Design review of the part built by this model. Coordinates are the model's own, in mm. A direction names the side the tool comes from. Coordinates: 2 decimals unless noted, no trailing zeros. Loops run counter-clockwise (first coordinate to the right, second up) from the corner with the lowest first, then second, coordinate; pieces in that order, holes last. Notation, with made-up numbers: (47.25, -30.75) -> (95.25, -30.75) arc R16 cw to (95.25, -7.75) -> close; hole circle Ø1 at (-33.5, -23). An arc over 180 degrees is marked (long way). Answer as a JSON object with one key per item and string values.
```python
from build123d import *

# Parameters (mm, degrees)
SKETCH1_W           = 7.5
SKETCH1_H           = 6
BOSS_EXTRUDE1_DEPTH = 3


with BuildPart() as part:
    # Sketch1 → Boss-Extrude1 (new body)
    with BuildSketch(Plane(origin=(0, 0, 0), x_dir=(1, 0, 0), z_dir=(0, 1, 0))):
        Polygon((0, 0), (0, 25.5), (-7.5, 25.5), (-15, 25.5), (-15, -12.75), (0, -12.75), align=None)
        Polygon((0, -25.5), (0, -12.75), (-15, -12.75), (-15, -25.5), (-7.5, -25.5), align=None)
        Polygon((15, -12.75), (0, -12.75), (0, -25.5), (7.5, -25.5), (15, -25.5), align=None)
        Polygon((7.5, 25.5), (0, 25.5), (0, 0), (0, -12.75), (15, -12.75), (15, 25.5), align=None)
        Polygon((-7.5, 25.5), (0, 25.5), (7.5, 25.5), (7.5, 28.5), (-7.5, 28.5), align=None)
        Polygon((-7.5, 25.5), (0, 25.5), (7.5, 25.5), (7.5, 28.5), (-7.5, 28.5), align=None)
        with Locations((-3.75, -28.5)):
            Rectangle(SKETCH1_W, SKETCH1_H)
        with Locations((3.75, -28.5)):
            Rectangle(SKETCH1_W, SKETCH1_H)
    extrude(amount=BOSS_EXTRUDE1_DEPTH)


solid = part.part
```
1) Add section A-A, the plane y = 1.75. Give the boundary of the cut face in (x, z).
Completed:
{"outline": "(-15, -25.5) -> (-7.5, -25.5) -> (-7.5, -28.5) -> (7.5, -28.5) -> (7.5, -25.5) -> (15, -25.5) -> (15, 25.5) -> (7.5, 25.5) -> (7.5, 31.5) -> (-7.5, 31.5) -> (-7.5, 25.5) -> (-15, 25.5) -> close"}
2) Clearance check with flat-ended pins moving along their axes: pin 1 Ø0.9 at (x, y) = (10.5, 1.5) entering from +Z; pin 2 Ø1.5 at (x, y) = (-12.5, 1.5) entering from -Z; pin 3 Ø0.9 at (y, z) = (2, -26.5) entering from +X. State where each tip first meets the part, or that it passes through.
Completed:
{"pin 1": "z = 25.5", "pin 2": "z = -25.5", "pin 3": "x = 7.5"}
3) Add section B-B, the plane x = -10.5. Give the boundary of the cut face in (y, z).
Completed:
{"outline": "(0, -25.5) -> (3, -25.5) -> (3, 25.5) -> (0, 25.5) -> close"}
4) Wall thickness on probe 1 along Z at (x, y) = (-12.5, 1.55); probe 2 along X at (y, z) = (1.6, 28.5): over which ranges is each line inside the solid? List them lowest first.
Completed:
{"probe 1": "-25.5 to 25.5", "probe 2": "-7.5 to 7.5"}
5) For faces 1 (the flat face through (-11, 1, -25.5)), 2 (the flat face through (-11, 1, 25.5)), 3 (the flat face through (11, 1, 25.5)), 4 (the flat face through (11, 1, -25.5)), list the 3-axis set-ups (+Z, -Z, +X, -X, +Y, -Y) from which the entire face can be reached by the end or side of a thin tool; tool diameter is ignored.
Completed:
{"face 1": "-Z, -X, +Y, -Y", "face 2": "+Z, -X, +Y, -Y", "face 3": "+Z, +X, +Y, -Y", "face 4": "-Z, +X, +Y, -Y"}
